from build123d import *

# Parameters (mm, degrees)
SKETCH1_W                                = 70
SKETCH1_H                                = 100
BOSS_EXTRUDE1_DEPTH                      = 5
SKETCH3_R                                = 2.5
BOSS_EXTRUDE2_DEPTH                      = 20
CBORE_FOR_1_4_HEX_HEAD_BOLT1_D           = 7.14248
CBORE_FOR_1_4_HEX_HEAD_BOLT1_CBORE_D     = 19.05
CBORE_FOR_1_4_HEX_HEAD_BOLT1_CBORE_DEPTH = 4.7752
CIRPATTERN2_COUNT                        = 2
SKETCH8_R                                = 1.5
CUT_EXTRUDE2_DEPTH                       = 10


with BuildPart() as part:
    # Sketch1 → Boss-Extrude1 (new, symmetric)
    with BuildSketch(Plane.XY):
        Rectangle(SKETCH1_W, SKETCH1_H)
    extrude(amount=BOSS_EXTRUDE1_DEPTH, both=True)

    # Sketch3 → Boss-Extrude2 (add)
    with BuildSketch(Plane.XY.offset(5)):
        with Locations(Location((0, 0, 0), (0, 0, 180))):
            Circle(SKETCH3_R)
    extrude(amount=BOSS_EXTRUDE2_DEPTH)

    # Sketch5 → Revolve1 (revolve)
    with BuildSketch(Plane(origin=(0, 0, 0), x_dir=(0, 0, -1), z_dir=(1, 0, 0))):
        Polygon((-5, 6), (-15, 6), (-15, 8), (-25, 8), (-25, 10), (-5, 10), align=None)
    revolve(axis=Axis((0, 0, 0), (0, 0, 1)))

    # CBORE for 1/4 Hex Head Bolt1 (through all)
    with Locations(Plane(origin=(0, 30, 5), x_dir=(1, 0, 0), z_dir=(0, 0, 1))):
        with Locations((0, 0)):
            cbore_for_1_4_hex_head_bolt1 = CounterBoreHole(CBORE_FOR_1_4_HEX_HEAD_BOLT1_D / 2, CBORE_FOR_1_4_HEX_HEAD_BOLT1_CBORE_D / 2, CBORE_FOR_1_4_HEX_HEAD_BOLT1_CBORE_DEPTH)

    # CirPattern2: CBORE for 1/4 Hex Head Bolt1 ×2 about axis
    cirpattern2_axis = Axis((0, 0, 0), (0, 0, 1))
    for i in range(1, CIRPATTERN2_COUNT):
        add(cbore_for_1_4_hex_head_bolt1.rotate(cirpattern2_axis, i * 360 / CIRPATTERN2_COUNT), mode=Mode.SUBTRACT)

    # Sketch8 → Cut-Extrude2 (cut)
    with BuildSketch(Plane(origin=(-5, 0, 0), x_dir=(0, 0, -1), z_dir=(1, 0, 0))):
        with Locations((-14.239336727, 0)):
            Circle(SKETCH8_R)
    extrude(amount=-CUT_EXTRUDE2_DEPTH, mode=Mode.SUBTRACT)


solid = part.part
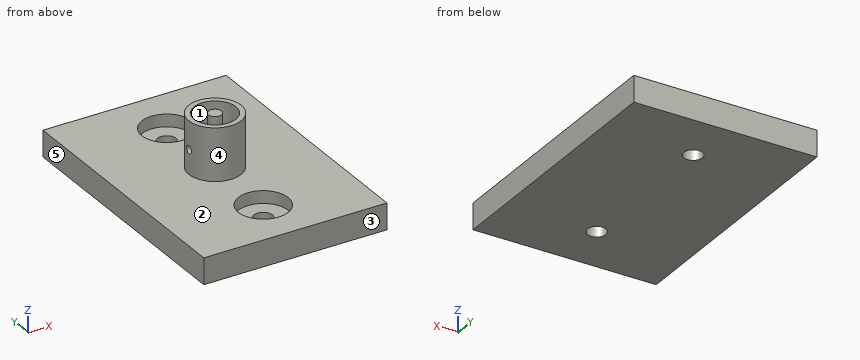
Check sheet for the modelled part. Datum: model origin and axes. Units: mm. Face numbers are marked on the shaded views. A direction names the side the tool comes from. Round coordinates to 2 decimals unless told otherwise and drop trailing zeros. Loops run counter-clockwise (first coordinate to the right, second up) from the corner with the lowest first, then second, coordinate; pieces in that order, holes last. Notation, with made-up numbers: (77, 49.25) - (127, 49.25) arc R22 cw to (127, 79.25) - close; hole circle Ø7 at (-29, -2). An arc over 180 degrees is marked (long way). Answer as CSV lines item,"result". Start each with the question number.
Item 1: Section check A-A (y = 30). Record the boundary of the cut face in (x, z) (3 decimals).
Item 2: Section check B-B (z = 9.5). Record the boundary of the cut face in (x, y), and give its area (3 significant figures).
Item 3: Set-up check for the marked faces 4 and 5: record each of +Z, -Z, +X, -X, +Y, -Y from which the full face is reachable in a straight line by a thin tool's end or side.
Item 4: Scan lines: line 1 (Y direction, x = 0, z = 2.4) (3 decimals); line 2 (Y direction, x = 0, z = -0.85); line 3 (Z direction, x = -9.1, y = 0). Record each from-to range of solid material in increasing order. Write a range as [from, to].
Item 5: Section check C-C (y = 0). Record the boundary of the cut face in (x, z).
Item 6: Release check for a two-part mould opening along Y. For the marked faces 1, 2 and 3 record: +Y half, -Y half, draft (parallel to the pull), parting line (faces both ways), or undercut.
Item 7: Depth check by flat-ended pin: P1, Ø5, axis at y = 14, z = 5.5, coming from the +X side; P2, Ø22, axis at x = 0, y = 30, coming from the +Z side; P3, Ø9.5, axis at x = 0, y = 30, coming from the +Z side; P4, Ø8, axis at x = -1.5, z = 11.5, coming from the +Y side. Enter the tip coordinate at first touch or a pass-through.
Item 8: Section check D-D (z = 2.5). Record the boundary of the cut face in (x, y) (3 decimals).
Report:
1,outline,"(-35, -5) - (-3.571, -5) - (-3.571, 0.225) - (-9.525, 0.225) - (-9.525, 5) - (-35, 5) - close; (3.571, -5) - (35, -5) - (35, 5) - (9.525, 5) - (9.525, 0.225) - (3.571, 0.225) - close"
2,outline,"circle Ø20 at (0, 0); circle Ø5 at (0, 0); hole circle Ø12 at (0, 0)"
2,area,"221 mm2"
3,face 4,"+Z"
3,face 5,"+Z, -Z, -X, +Y, -Y"
4,line 1,"y = [-50, -39.525], [-20.475, 20.475], [39.525, 50]"
4,line 2,"y = [-50, -33.57], [-26.43, 26.43], [33.57, 50]"
4,line 3,"z = [-5, 12.74], [15.74, 25]"
5,outline,"(-35, -5) - (35, -5) - (35, 5) - (10, 5) - (10, 25) - (8, 25) - (8, 15) - (6, 15) - (6, 5) - (2.5, 5) - (2.5, 25) - (-2.5, 25) - (-2.5, 5) - (-6, 5) - (-6, 12.74) - (-10, 12.74) - (-10, 5) - (-35, 5) - close; (-10, 15.74) - (-8, 15.74) - (-8, 25) - (-10, 25) - close"
6,face 1,"undercut"
6,face 2,"draft"
6,face 3,"-Y half"
7,P1,"stops at x = 35"
7,P2,"stops at z = 5"
7,P3,"stops at z = 0.22"
7,P4,"stops at y = 10"
8,outline,"(-35, -50) - (35, -50) - (35, 50) - (-35, 50) - close; hole circle Ø19.05 at (0, -30); hole circle Ø19.05 at (0, 30)"
